Print and shaded views of the part. All mm, measured from the part's lowest x, y and z. A direction names the side the tool comes from. Coordinates: 2 decimals unless noted, no trailing zeros. Loops run counter-clockwise (first coordinate to the right, second up) from the corner with the lowest first, then second, coordinate; pieces in that order, holes last. Notation, with made-up numbers: M 71,2.25 L 79,2.25 A29 cw 79,23.25 Z; hole C 76,19.25 d9. An arc over 180 degrees is marked long. Answer as a JSON object with one key per item and string values. Group by question number.
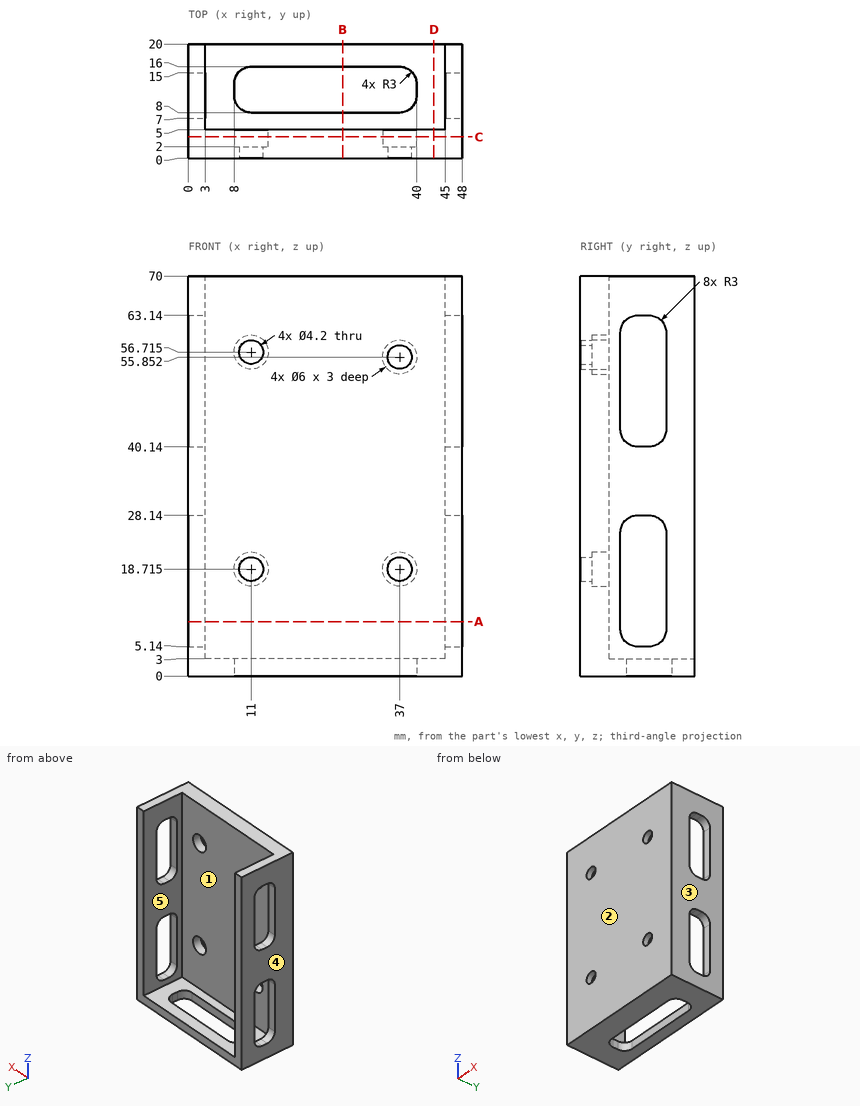
Item 1: Slice it at C-C, the plane y = 3.75. Write the cut outline in (x, z) (1 decimal), then the cut area to 3 significant figures.
Item 2: Slice it at A-A, the plane z = 9.5. Write the cut outline in (x, y).
Item 3: Drill centre lines: L1, parallel to Z at x = 11, y = 2.75 (1 decimal); L2, parallel to Z at x = 11, y = 1.5 (1 decimal); L3, parallel to X at y = 16.75, z = 13.5. Where is each one in solid material? Low to high. Write a range as from..to.
Item 4: Slice it at D-D, the plane x = 43. Write the cut outline in (y, z), then the cut area to 3 significant figures.
Item 5: Pull direction X, two halves, no side cores. Call the marked faces 1, 2 and 3: released by +X, released by -X, zero draft, split by the parting line, or undercut.
Item 6: Slice it at B-B, the plane x = 27. Write the cut outline in (y, z), then the cut area to 3 significant figures.
Item 7: Tool access for the marked faces 4 and 5: list every direction of +Z, -Z, +X, -X, +Y, -Y with a clear straight run to the whole face (end or side of a thin tool).
Item 8: Pin check, flat tips, straight feed: pin 1 (7.5 mm diameter, centred on x = 31, y = 9.5, fed in from +Z); pin 2 (1.5 mm diameter, centred on x = 8, z = 26.5, fed in from +Y). Stop position of each tip, or through.
Computed:
{
 "1": {"outline": "M 0,0 L 48,0 L 48,70 L 0,70 Z; hole C 11,18.7 d6; hole C 11,56.7 d6; hole C 37,18.7 d6; hole C 37,55.9 d6", "area": "3,250 mm2"},
 "2": {"outline": "M 0,0 L 48,0 L 48,7 L 45,7 L 45,5 L 3,5 L 3,7 L 0,7 Z; M 0,15 L 3,15 L 3,20 L 0,20 Z; M 45,15 L 48,15 L 48,20 L 45,20 Z"},
 "3": {"L1": "0..15.7, 21.7..53.7, 59.7..70", "L2": "0..16.6, 20.8..54.6, 58.8..70", "L3": "0..3, 45..48"},
 "4": {"outline": "M 0,0 L 20,0 L 20,3 L 5,3 L 5,70 L 0,70 Z", "area": "395 mm2"},
 "5": {"face 1": "undercut", "face 2": "zero draft", "face 3": "released by +X"},
 "6": {"outline": "M 0,0 L 8,0 L 8,3 L 5,3 L 5,70 L 0,70 Z; M 16,0 L 20,0 L 20,3 L 16,3 Z", "area": "371 mm2"},
 "7": {"face 4": "+Z, -Z, -X, +Y, -Y", "face 5": "+Z, +Y"},
 "8": {"pin 1": "z = 3", "pin 2": "y = 5"}
}
